Read the model definition and answer for the solid it produces. Units are mm, in the model's axes. Face numbers are marked on the shaded views. A direction names the side the tool comes from. Coordinates: 2 decimals unless noted, no trailing zeros. Order: outer loops, then holes, each group sorted by start corner. A loop starts at its lowest first (then second) coordinate and runs counter-clockwise, first axis right, second up. Notation, with made-up numbers: M 23,34.25 L 78,34.25 A9 cw 78,39.25 Z; hole C 19.25,-33.75 d5. An arc over 180 degrees is marked long. One line per question, with ' | ' between items. Start each with the question number.
1) Find section B-B, the plane z = 1. Write down the section's boundary in (x, y).
2) Find section D-D, the plane z = 6.5. Write down the section's boundary in (x, y).
3) Consider probe 1 along Y at (x, z) = (-8, 5); probe 2 along Y at (x, z) = (20, 7.75); probe 3 along X at (y, z) = (4, 1.75). Determine where each line is inside the solid, lowest interval first.
4) The mould has two halves that part along Z. Classify the marked faces 1, 2 and 3: +Z half, -Z half, draft (parallel to the pull), parting line (faces both ways), or undercut.
5) Find section A-A, the plane y = 4. Write down the section's boundary in (x, z).
6) A tool of negligible diameter and unlimited length cuts with its end or side. For the marked faces 4, 5 and 6, from which of +Z, -Z, +X, -X, +Y, -Y can it reach the whole face along a straight path? Write none if from no direction.
7) Find section C-C, the plane x = 20. Write down the section's boundary in (y, z), plus the area to 3 significant figures.
8) Given P1, Ø3, axis at x = -0.5, z = 8, coming from the -Y side; P2, Ø3, axis at y = 0.5, z = 4.5, coming from the -X side; P3, Ø3, axis at x = -6, z = 4, coming from the +Y side; P4, Ø13, axis at x = 20, y = 0, coming from the +Z side, each flat-ended and moving along its own axis, determine where each tip first touches the part or whether it passes through.
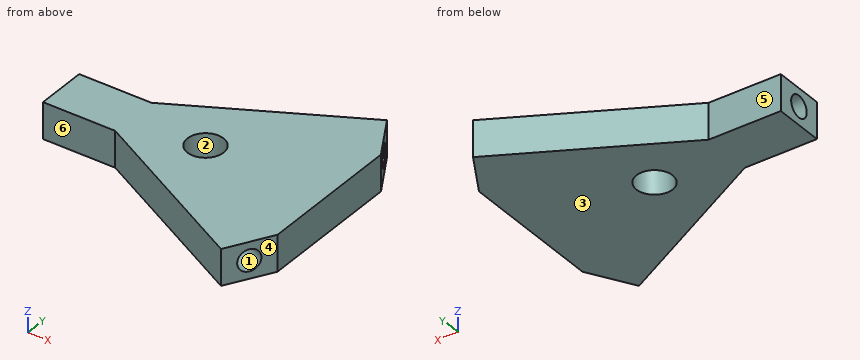
from build123d import *

# Parameters (mm, degrees)
BOSS_EXTRU_2_DEPTH      = 10
ESQUISSE4_R             = 3
ENL_V_MAT_EXTRU_3_DEPTH = 20
ESQUISSE6_R             = 3
ENL_V_MAT_EXTRU_4_DEPTH = 20
ESQUISSE7_R             = 3
ENL_V_MAT_EXTRU_5_DEPTH = 20
ESQUISSE8_R             = 5
ENL_V_MAT_EXTRU_6_DEPTH = 20


with BuildPart() as part:
    # Esquisse1 → Boss.-Extru.2 (new body)
    with BuildSketch(Plane.XY):
        Polygon((-20, -7), (-20, 7), (0, 7), (47.282032303, 32.124355653), (54.282032303, 20), (54.282032303, -20), (47.282032303, -32.124355653), (0, -7), align=None)
    extrude(amount=BOSS_EXTRU_2_DEPTH)

    # Esquisse4 → Enlèv. mat.-Extru.3 (cut)
    with BuildSketch(Plane.ZY.offset(20)):
        with Locations((5, 0)):
            Circle(ESQUISSE4_R)
    extrude(amount=-ENL_V_MAT_EXTRU_3_DEPTH, mode=Mode.SUBTRACT)

    # Esquisse6 → Enlèv. mat.-Extru.4 (cut)
    with BuildSketch(Plane(origin=(49.371778265, 28.504809472, 0), x_dir=(0.4999999999999953, -0.8660254037844415, 0), z_dir=(0.8660254037844415, 0.4999999999999953, 0))):
        with Locations(Location((2.820508076, -5, 0), (0, 0, 180))):
            Circle(ESQUISSE6_R)
    extrude(amount=-ENL_V_MAT_EXTRU_4_DEPTH, mode=Mode.SUBTRACT)

    # Esquisse7 → Enlèv. mat.-Extru.5 (cut)
    with BuildSketch(Plane(origin=(49.371778265, -28.504809472, 0), x_dir=(-0.5000000000000256, -0.8660254037844237, 0), z_dir=(0.8660254037844238, -0.5000000000000258, 0))):
        with Locations(Location((-2.820508076, -5, 0), (0, 0, 180))):
            Circle(ESQUISSE7_R)
    extrude(amount=-ENL_V_MAT_EXTRU_5_DEPTH, mode=Mode.SUBTRACT)

    # Esquisse8 → Enlèv. mat.-Extru.6 (cut)
    with BuildSketch(Plane(origin=(0, 0, 0), x_dir=(-1, 0, 0), z_dir=(0, 0, -1))):
        with Locations((-20, 0)):
            Circle(ESQUISSE8_R)
    extrude(amount=-ENL_V_MAT_EXTRU_6_DEPTH, mode=Mode.SUBTRACT)


solid = part.part
Report:
1) outline: M -20,-7 L 0,-7 L 47.28,-32.12 L 54.28,-20 L 54.28,20 L 47.28,32.12 L 0,7 L -20,7 Z; hole C 20,0 d10
2) outline: M -20,-7 L 0,-7 L 47.28,-32.12 L 49.48,-28.31 L 32.16,-18.31 L 34.76,-13.81 L 52.08,-23.81 L 54.28,-20 L 54.28,20 L 52.08,23.81 L 34.76,13.81 L 32.16,18.31 L 49.48,28.31 L 47.28,32.12 L 0,7 L -20,7 L -20,2.6 L 0,2.6 L 0,-2.6 L -20,-2.6 Z; hole C 20,0 d10
3) probe 1: y = -7 to -3, 3 to 7 | probe 2: y = -17.63 to -5, 5 to 17.63 | probe 3: x = -20 to 17, 23 to 54.28
4) face 1: undercut | face 2: draft | face 3: -Z half
5) outline: M -20,0 L 17,0 L 17,10 L -20,10 Z; M 23,0 L 54.28,0 L 54.28,10 L 23,10 Z
6) face 4: +Z, -Z, +X, -Y | face 5: +Z, -Z, -X, +Y | face 6: +Z, -Z, -X, -Y
7) outline: M -17.63,0 L -5,0 L -5,10 L -17.63,10 Z; M 5,0 L 17.63,0 L 17.63,10 L 5,10 Z | area: 253 mm^2
8) P1: stops at y = -7.53 | P2: stops at x = 0 | P3: stops at y = 7 | P4: stops at z = 10
